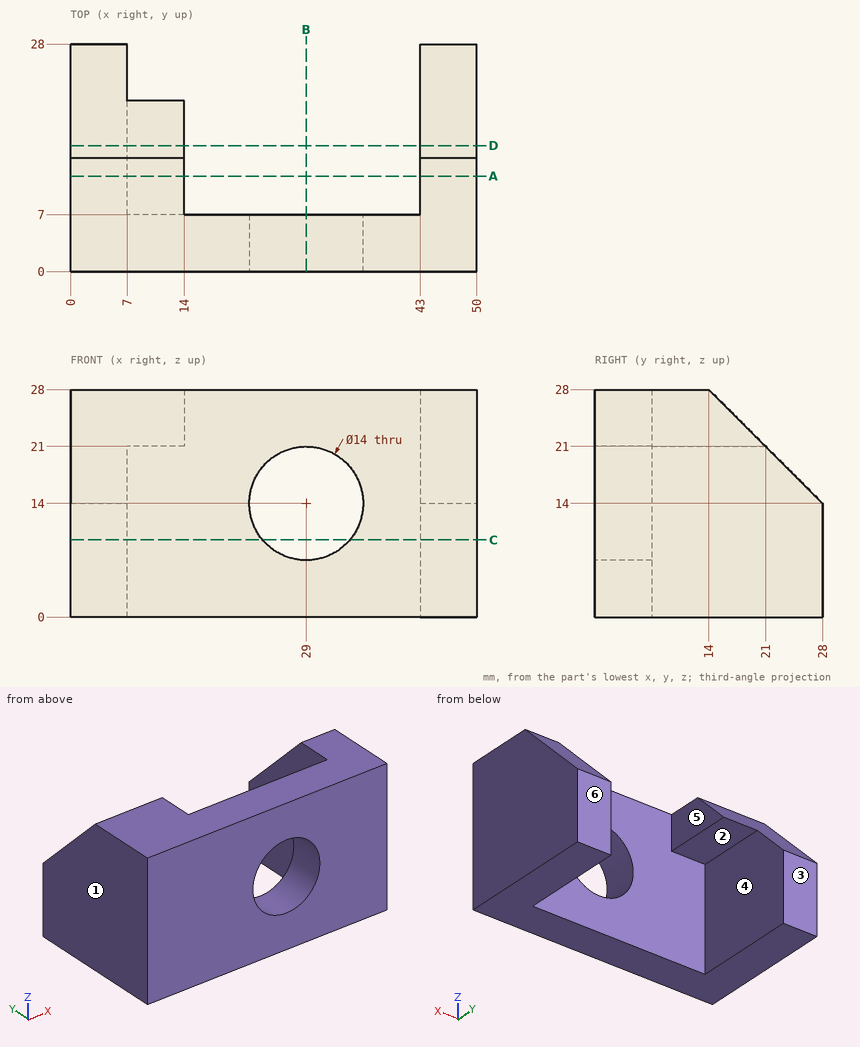
Source: three-view drawing plus pictorial views. Frame: mm from the lowest corner of the part. A direction names the side the tool comes from. Coordinates: 2 decimals unless noted, no trailing zeros. Loops run counter-clockwise (first coordinate to the right, second up) from the corner with the lowest first, then second, coordinate; pieces in that order, holes last. Notation, with made-up numbers: (24.5, 0) - (38.5, 0) arc R11 cw to (38.5, 17) - close; hole circle Ø8 at (18.5, 27.5). An arc over 180 degrees is marked (long way). One line per item, written item: value. Start each with the question number.
1. Set-up query: the marked faces 4, 5 and 6. Return all of +Z, -Z, +X, -X, +Y, -Y with unobstructed straight access to the full face (end or side cutting, diameter ignored); none if empty.
2. Mould query, pull axis X, two halves, no side actions, for the marked faces 1, 2 and 3. Classes: pulls with the +X half, pulls with the -X half, needs draft (parallel to the pull), parting line crosses it, or undercut.
3. Section A-A (y = 11.75). Return the cut outline in (x, z).
4. Contact query for flat-ended pins moving along their axis: P1, Ø3.5, axis at x = 11.5, y = 16.5, coming from the -Z side; P2, Ø12.5, axis at x = 29, z = 14, coming from the -Y side; P3, Ø8.5, axis at x = 31, z = 19, coming from the +Y side; P4, Ø4, axis at x = 15.5, z = 24.5, coming from the +Y side. Output: stop coordinate, or through.
5. Ray query, L1, parallel to X at y = 4, z = 14; L2, parallel to Z at x = 29, y = 2.75; L3, parallel to X at y = 16.75, z = 4.5. Return the intervals inside material, ascending.
6. Section B-B (x = 29). Return the cut outline in (y, z).
7. Section C-C (z = 9.5). Return the cut outline in (x, y), and give its area (3 significant figures).
8. Section D-D (y = 15.5). Return the cut outline in (x, z).
Verdict:
1. face 4: -Z, +Y
1. face 5: +Z, -Z, +Y
1. face 6: +Z, -Z, +X, -X, +Y
2. face 1: pulls with the -X half
2. face 2: undercut
2. face 3: needs draft
3. outline: (0, 0) - (7, 0) - (7, 21) - (14, 21) - (14, 28) - (0, 28) - close; (43, 0) - (50, 0) - (50, 28) - (43, 28) - close
4. P1: stops at z = 21
4. P2: passes through
4. P3: stops at y = 7
4. P4: stops at y = 18.82
5. L1: x = 0 to 22, 36 to 50
5. L2: z = 0 to 7, 21 to 28
5. L3: x = 0 to 7, 43 to 50
6. outline: (0, 0) - (7, 0) - (7, 7) - (0, 7) - close; (0, 21) - (7, 21) - (7, 28) - (0, 28) - close
7. outline: (0, 0) - (23.64, 0) - (23.64, 7) - (7, 7) - (7, 28) - (0, 28) - close; (34.36, 0) - (50, 0) - (50, 28) - (43, 28) - (43, 7) - (34.36, 7) - close
7. area: 569 mm2
8. outline: (0, 0) - (7, 0) - (7, 21) - (14, 21) - (14, 26.5) - (0, 26.5) - close; (43, 0) - (50, 0) - (50, 26.5) - (43, 26.5) - close
